Source: CAD feature listing. Evaluate the final solid. Frame: model axes, mm. A direction names the side the tool comes from. Give positions to 0.01 mm unless a question says otherwise; leave off trailing zeros. Write item = value, one per line.
from build123d import *

# Parameters (mm, degrees)
SKETCH1_R           = 2.286
BOSS_EXTRUDE1_DEPTH = 12.7
FILLET1_R           = 1.27
SKETCH2_R           = 4.445
CUT_EXTRUDE1_DEPTH  = 3.96875
SKETCH3_R           = 1.905
CUT_EXTRUDE2_DEPTH  = 12.7
SKETCH4_R           = 1.905
CUT_EXTRUDE3_DEPTH  = 12.7


with BuildPart() as part:
    # Sketch1 → Boss-Extrude1 (new body)
    with BuildSketch(Plane.XY):
        with BuildLine():
            Line((0.048604687, -6.34981398), (-101.551395313, -7.127511762))
            Line((-101.551395313, -7.127511762), (-129.54, -0.455968887))
            Line((-129.54, -0.455968887), (-200.976985186, -9.797318323))
            ThreePointArc((-200.976985186, -9.797318323), (-210.850504728, -8.14047549), (-218.115352674, -1.251825358))
            ThreePointArc((-218.115352674, -1.251825358), (-224.036255837, 6.613973279), (-231.775, 12.7))
            Line((-231.775, 12.7), (-218.115352674, 33.3375))
            Line((-218.115352674, 33.3375), (-202.035751798, 38.1))
            Line((-202.035751798, 38.1), (-133.35, 25.4))
            Line((-133.35, 25.4), (-128.905, 34.925))
            Line((-128.905, 34.925), (-79.17262462, 25.4))
            Line((-79.17262462, 25.4), (1.47237538, 6.17694186))
            ThreePointArc((1.47237538, 6.17694186), (6.309377787, -0.717113616), (0.048604687, -6.34981398))
        make_face()
        Circle(SKETCH1_R, mode=Mode.SUBTRACT)
        with Locations((-203.2, 7.20295315)):
            Circle(SKETCH1_R, mode=Mode.SUBTRACT)
    extrude(amount=BOSS_EXTRUDE1_DEPTH)

    # Fillet1
    fillet1_edges = [part.edges().sort_by_distance(p)[0] for p in [
        (-50.751395313, -6.738662871, 0),
        (-115.545697656, -3.791740325, 0),
        (-104.03881231, 30.1625, 12.7),
        (-165.258492593, -5.126643605, 0),
        (-210.850504728, -8.14047549, 0),
        (-224.036255837, 6.613973279, 0),
        (-224.945176337, 23.01875, 0),
        (-210.075552236, 35.71875, 0),
        (-167.692875899, 31.75, 0),
        (-131.1275, 30.1625, 0),
        (-104.03881231, 30.1625, 0),
        (-38.85012462, 15.78847093, 0),
        (6.309377787, -0.717113616, 0),
        (-131.1275, 30.1625, 12.7),
        (-167.692875899, 31.75, 12.7),
        (-231.775, 12.7, 6.35),
        (-128.905, 34.925, 6.35),
        (-210.075552236, 35.71875, 12.7),
        (-224.945176337, 23.01875, 12.7),
        (-224.036255837, 6.613973279, 12.7),
        (-210.850504728, -8.14047549, 12.7),
        (-165.258492593, -5.126643605, 12.7),
        (-115.545697656, -3.791740325, 12.7),
        (-50.751395313, -6.738662871, 12.7),
        (6.309377787, -0.717113616, 12.7),
        (-38.85012462, 15.78847093, 12.7),
    ]]
    fillet(fillet1_edges, radius=FILLET1_R)

    # Sketch2 → Cut-Extrude1 (cut)
    with BuildSketch(Plane(origin=(0, 0, 0), x_dir=(-1, 0, 0), z_dir=(0, 0, -1))):
        Circle(SKETCH2_R)
    extrude(amount=-CUT_EXTRUDE1_DEPTH, mode=Mode.SUBTRACT)

    # Sketch3 → Cut-Extrude2 (cut)
    with BuildSketch(Plane(origin=(0.132942268, 0.718995244, 0), x_dir=(0.9833321660356336, -0.18181818181818188, 0), z_dir=(0.18181818181818188, 0.9833321660356336, 0))):
        with Locations(Location((-179.556061292, -6.35, 0), (0, 0, 180))):
            Circle(SKETCH3_R)
        with Locations(Location((-141.456061292, -6.35, 0), (0, 0, 180))):
            Circle(SKETCH3_R)
    extrude(amount=-CUT_EXTRUDE2_DEPTH, mode=Mode.SUBTRACT)

    # Sketch4 → Cut-Extrude3 (cut)
    with BuildSketch(Plane(origin=(-167.013671414, 110.543808611, 0), x_dir=(0, 0, 1), z_dir=(-0.8338861185572083, 0.5519365373642097, 0))):
        with Locations(Location((6.35, -110.945024644, 0), (0, 0, 270))):
            Circle(SKETCH4_R)
    extrude(amount=-CUT_EXTRUDE3_DEPTH, mode=Mode.SUBTRACT)


solid = part.part
1) Contact query for flat-ended pins moving along their axis: pin 1 (5 mm diameter, centred on x = -131.5, z = 2.5, fed in from +Y); pin 2 (5 mm diameter, centred on x = -65, z = 11, fed in from +Y); pin 3 (1.5 mm diameter, centred on x = -34.5, z = 2, fed in from +Y). Output: stop coordinate, or through.
Computed:
pin_1 = 34.45
pin_2 = 22.62
pin_3 = 14.93
2) Draft query along X for faces 6 (the cylindrical face through (-115.773, -3.365, 12.318)), 7 (the cylindrical face through (-209.86, 35.405, 0.382)), 8 (the flat face through (-39.41, 15.92, 6.28)). Return one class per face: pulls with the +X half, pulls with the -X half, needs draft (parallel to the pull), parting line crosses it, or undercut.
Computed:
face_6 = undercut
face_7 = pulls with the -X half
face_8 = pulls with the +X half
3) Material intervals for L1, parallel to X at y = 0.5, z = 6.5; L2, parallel to X at y = 0, z = 6.5; L3, parallel to Y at x = 0, z = 8.75, sorted ascending.
Computed:
L1 = -219.17 to -2.23, 2.23 to 6.33
L2 = -218.86 to -2.29, 2.29 to 6.35
L3 = -6.35 to -2.29, 2.29 to 6.53
4) Access query for faces 1 (the flat face through (-141.248, 13.945, 6.377)), 2 (the flat face through (-115.35, -3.84, 6.28)), 3 (the cylindrical face through (-131.185, 29.183, 12.318)), 4 (the flat face through (-168.17, 31.84, 6.28)), 5 (the cylindrical face through (-165.691, -4.818, 0.382)). Directions: +Z, -Z, +X, -X, +Y, -Y. A direction counts if a zero-diameter tool reaches every point of the face in a straight line with its end or side. Return the directions, or none.
Computed:
face_1 = none
face_2 = +Z, -Z, -Y
face_3 = +Z, +Y
face_4 = +Z, -Z, +Y
face_5 = -Z, -Y
